Geometry: see drawing. Coordinates: mm, zero at the bounding-box minimum. Coordinates: 2 decimals unless noted, no trailing zeros. Write each loop counter-clockwise with the first axis right and the second up, starting at its lowest first coordinate (ties: lowest second). Pieces come first, ordered by that corner, then holes. Notation, with made-up numbers: (-8.75, 18) -> (25.25, 18) arc R19 ccw to (25.25, 42) -> close; hole circle Ø8 at (-8.5, 62). An arc over 180 degrees is marked (long way). Use one line per item in the form item = value. Start each with the question number.
(1) First-contact query: pin 1 (3 mm diameter, centred on x = 78.46, z = 13.52, fed in from +Y). Flat tip, straight axial feed; report the tip coordinate or a pass-through.
(2) Cut plane A-A on x = 22. Return the cut outline in (y, z), plus the area to 3 significant figures.
(3) Ray query, line 1 along Z through (x, y) = (22, 3.4); line 2 along X through (y, z) = (0.3, 13.5); line 3 along X through (y, z) = (2.1, 91). Return the intervals inside material, ascending.
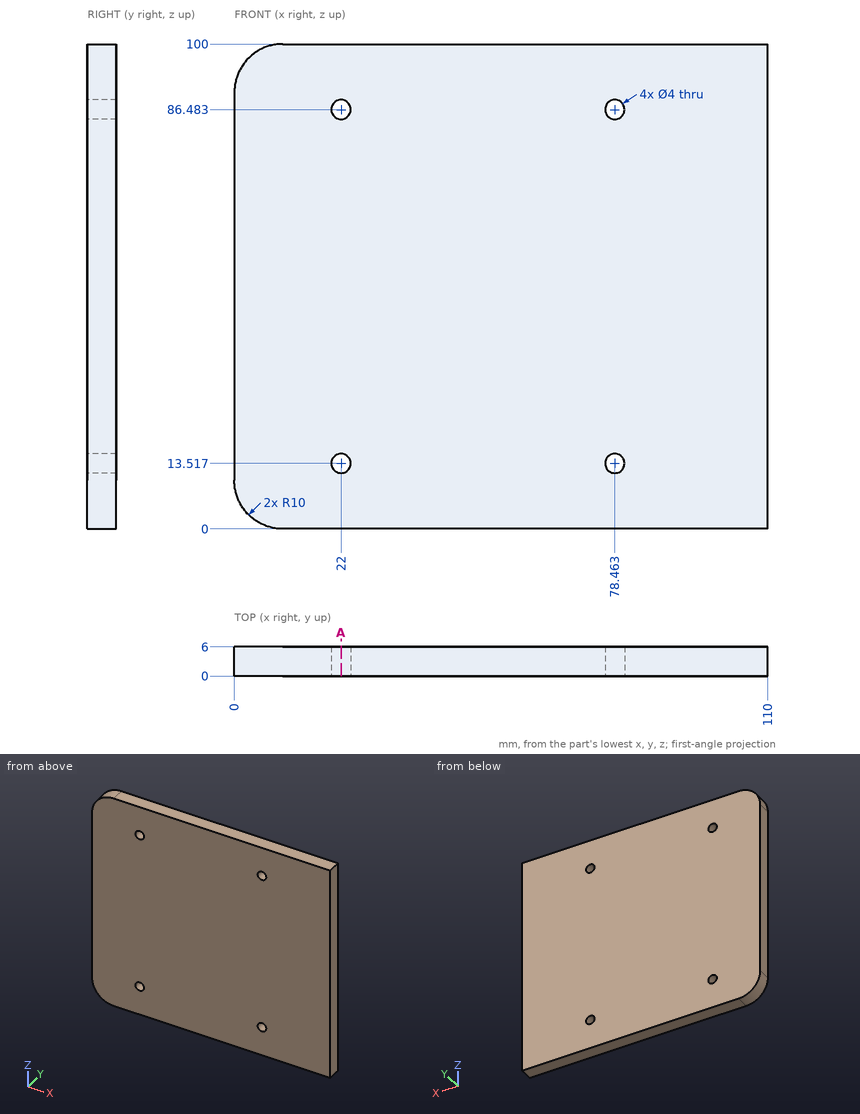
Values:
q1.pin_1 = through
q2.outline = (0, 0) -> (6, 0) -> (6, 11.52) -> (0, 11.52) -> close; (0, 15.52) -> (6, 15.52) -> (6, 84.48) -> (0, 84.48) -> close; (0, 88.48) -> (6, 88.48) -> (6, 100) -> (0, 100) -> close
q2.area = 552 mm2
q3.line_1 = 0 to 11.52, 15.52 to 84.48, 88.48 to 100
q3.line_2 = 0 to 20, 24 to 76.46, 80.46 to 110
q3.line_3 = 0.05 to 110
